For this review, take the finished solid that the model builds, in its own axes (mm). Face numbers are marked on the shaded views. Coordinates: 2 decimals unless noted, no trailing zeros. Order: outer loops, then holes, each group sorted by start corner. A loop starts at its lowest first (then second) coordinate and runs counter-clockwise, first axis right, second up. Notation, with made-up numbers: M -32.5,49.5 L 18.5,49.5 A12 ccw 18.5,62.5 Z; hole C 79.25,21 d7. An arc over 180 degrees is marked long. Use CSV: the item, a comma, the result in double quotes.
```python
from build123d import *

# Parameters (mm, degrees)
F4_R     = 6.35
F4_R_2   = 3.81
F5_DEPTH = 2.54


with BuildPart() as f3:
    # F0 (on Top) → F3 section 0
    with BuildSketch(Plane.XY):
        with BuildLine():
            Line((0, 17.78), (0, 0))
            Line((0, 0), (5.08, 0))
            ThreePointArc((5.08, 0), (8.5405078821, 12.4809492118), (7.62, 25.4))
            ThreePointArc((7.62, 25.4), (2.2318463274, 23.1681536726), (0, 17.78))
        make_face()
    # F2 (on offset) → F3 section 1
    with BuildSketch(Plane.XY.offset(2.54)):
        Polygon((0, 19.05), (0, 0), (1.27, 0), (0.254, 19.05), align=None)
    loft()

    # F4 (on Top) → F5 (join, through all)
    with BuildSketch(Plane.XY):
        with Locations((2.54, -5.08)):
            Circle(F4_R)
        with Locations((2.54, -5.08)):
            Circle(F4_R_2, mode=Mode.SUBTRACT)
    extrude(amount=F5_DEPTH)


solid = f3.part
```
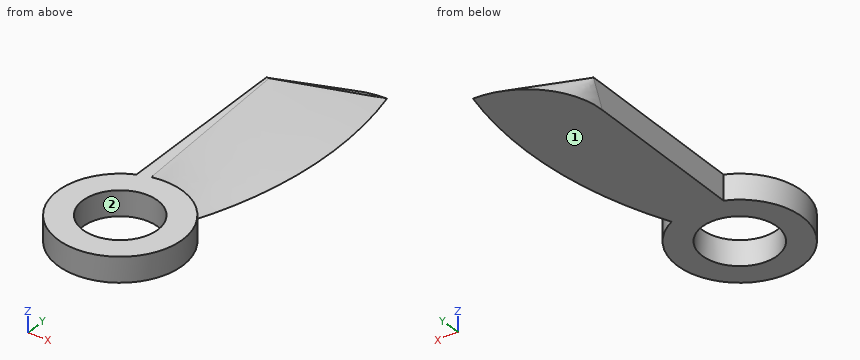
Item 1: Draft analysis for pull direction Y (two halves, no side actions). For the marked faces 1 and 2, state which applies: released by +Y, released by -Y, zero draft, split by the parting line, or undercut.
Solutions:
face 1,"zero draft"
face 2,"undercut"
Item 2: To check wall thickness, follow line 1 along Y through (x, z) = (2.54, 0.9); line 2 along Y through (x, z) = (5, 2.1); line 3 along X through (y, z) = (-6, 1.95). State the ranges of each line that lie inside material, in increasing order. Write a range as [from, to].
Solutions:
line 1,"[-11.43, -8.89], [-1.27, 22.5]"
line 2,"[-10.93, -7.99], [-2.17, 0.77]"
line 3,"[-3.74, -1.16], [6.24, 8.82]"
Item 3: Clearance check with flat-ended pins moving along their axes: pin 1 Ø2 at (x, y) = (0.5, 8.5) entering from -Z; pin 2 Ø1.5 at (y, z) = (4, 2) entering from +X. State where each tip first meets the part, or that it passes through.
Solutions:
pin 1,"z = 0"
pin 2,"x = 4.02"
Item 4: Add section B-B on x = 6. State how many separate pieces and enclosed holes the cut face has, and give its area (3 significant figures).
Solutions:
separate pieces,"3"
enclosed holes,"0"
area,"34.2 mm^2"
Item 5: Add section A-A on y = -5.08. State the section outline as (x, z) points.
Solutions:
outline,"M -3.81,0 L -1.27,0 L -1.27,2.54 L -3.81,2.54 Z; M 6.35,0 L 8.89,0 L 8.89,2.54 L 6.35,2.54 Z"
